from build123d import *

# Parameters (mm, degrees)
SKETCH_1_W             = 14
SKETCH_1_H             = 15
EXTRUDE_1_DEPTH        = 35
SKETCH_2_R             = 6
CUT_EXTRUDE_1_DEPTH    = 15
CUT_EXTRUDE_2_REACH    = 17
SKETCH_3_W             = 2
SKETCH_3_H             = 10
SKETCH_3_W_2           = 7
HOLE_WIZARD_M4_1_D     = 3.3
HOLE_WIZARD_M4_1_DEPTH = 5
SKETCH_4_R             = 4
CUT_EXTRUDE_3_DEPTH    = 1
FILLET_1_R             = 0.5


with BuildPart() as part:
    # 草图1 → 凸台-拉伸1 (new body)
    with BuildSketch(Plane.XY):
        with Locations((7, -7.5)):
            Rectangle(SKETCH_1_W, SKETCH_1_H)
    extrude(amount=EXTRUDE_1_DEPTH)

    # 草图2 → 切除-拉伸1 (cut)
    with BuildSketch(Plane.XY.offset(35)):
        with Locations((7, -7.5)):
            Circle(SKETCH_2_R)
    extrude(amount=-CUT_EXTRUDE_1_DEPTH, mode=Mode.SUBTRACT)

    # 草图3 → 切除-拉伸2 (cut, up to next)
    with BuildSketch(Plane.XZ.offset(15), mode=Mode.PRIVATE) as cut_extrude_2_sk1:
        with Locations((1, 5)):
            Rectangle(SKETCH_3_W, SKETCH_3_H)
    cut_extrude_2_tool1 = extrude(cut_extrude_2_sk1.sketch, amount=-CUT_EXTRUDE_2_REACH, mode=Mode.PRIVATE) & part.part
    add(cut_extrude_2_tool1.solids().sort_by_distance((1, -15, 5))[0], mode=Mode.SUBTRACT)
    # 草图3 → 切除-拉伸2 (cut, up to next)
    with BuildSketch(Plane.XZ.offset(15), mode=Mode.PRIVATE) as cut_extrude_2_sk2:
        with Locations((10.5, 5)):
            Rectangle(SKETCH_3_W_2, SKETCH_3_H)
    cut_extrude_2_tool2 = extrude(cut_extrude_2_sk2.sketch, amount=-CUT_EXTRUDE_2_REACH, mode=Mode.PRIVATE) & part.part
    add(cut_extrude_2_tool2.solids().sort_by_distance((10.5, -15, 5))[0], mode=Mode.SUBTRACT)

    # M4 螺纹孔1
    with Locations(Plane.ZY.offset(-2)):
        with Locations((5, -7.5)):
            Hole(HOLE_WIZARD_M4_1_D / 2, depth=HOLE_WIZARD_M4_1_DEPTH)

    # 草图4 → 切除-拉伸3 (cut)
    with BuildSketch(Plane.ZY.offset(-2)):
        with Locations((5, -7.5)):
            Circle(SKETCH_4_R)
    extrude(amount=-CUT_EXTRUDE_3_DEPTH, mode=Mode.SUBTRACT)

    # 圆角1
    fillet_1_edges = [part.edges().sort_by_distance(p)[0] for p in [
        (1, -7.5, 20),
        (1, -7.5, 35),
        (0, -7.5, 10),
        (14, -7.5, 10),
        (0, 0, 22.5),
        (14, 0, 22.5),
        (14, -15, 22.5),
        (0, -15, 22.5),
    ]]
    fillet(fillet_1_edges, radius=FILLET_1_R)


solid = part.part
Verification items for the finished model (mm, model axes). A direction names the side the tool comes from. Give positions to 0.01 mm unless a question says otherwise; leave off trailing zeros. Order: outer loops, then holes, each group sorted by start corner. A loop starts at its lowest first (then second) coordinate and runs counter-clockwise, first axis right, second up. Notation, with made-up numbers: (1.25, 70.25) -> (53.25, 70.25) arc R21 ccw to (53.25, 97.25) -> close; hole circle Ø10 at (64, 6.25). An arc over 180 degrees is marked (long way). Answer as CSV lines item,"result".
Q1. Sectioned sample at B-B on z = 24. Record the cut outline in (x, y), plus the area to 3 significant figures.
Solutions:
outline,"(0, -14.5) arc R0.5 ccw to (0.5, -15) -> (13.5, -15) arc R0.5 ccw to (14, -14.5) -> (14, -0.5) arc R0.5 ccw to (13.5, 0) -> (0.5, 0) arc R0.5 ccw to (0, -0.5) -> close; hole circle Ø12 at (7, -7.5)"
area,"96.7 mm²"
Q2. Release check for a two-part mould opening along Z. For faces 1 (the flat face through (3, -7, 7)), 2 (the flat face through (10, -8, 10)), 3 (the flat face through (7, 0, 21)) record: +Z half, -Z half, draft (parallel to the pull), parting line (faces both ways), or undercut.
Solutions:
face 1,"undercut"
face 2,"-Z half"
face 3,"draft"
Q3. Sectioned sample at A-A on y = -7.5. Record the cut outline in (x, z).
Solutions:
outline,"(0, 10.5) arc R0.5 ccw to (0.5, 10) -> (2, 10) -> (2, 9) -> (3, 9) -> (3, 6.65) -> (7, 6.65) -> (7, 10) -> (13.5, 10) arc R0.5 ccw to (14, 10.5) -> (14, 35) -> (13.5, 35) arc R0.5 ccw to (13, 34.5) -> (13, 20.5) arc R0.5 cw to (12.5, 20) -> (1.5, 20) arc R0.5 cw to (1, 20.5) -> (1, 34.5) arc R0.5 ccw to (0.5, 35) -> (0, 35) -> close; (2, 0) -> (7, 0) -> (7, 3.35) -> (3, 3.35) -> (3, 1) -> (2, 1) -> close"
Q4. Access from +Z, -Z, +X, -X, +Y, -Y to the whole of each face (thin tool, end or side, straight path). Record for faces 4 (the cylindrical face through (2.493, -6.299, 8.815)), 5 (the flat face through (7, -9.3, 4.9)), 6 (the flat face through (7, -7, 20)).
Solutions:
face 4,"-X"
face 5,"-Z, +X, +Y, -Y"
face 6,"+Z"
Q5. Depth check by flat-ended pin: pin 1 (4.5 mm diameter, centred on y = -7.5, z = 5, fed in from +X); pin 2 (1.7 mm diameter, centred on x = 1, y = -7, fed in from -Z); pin 3 (2.5 mm diameter, centred on y = -7, z = 6.5, fed in from -X). Enter the tip coordinate at first touch or a pass-through.
Solutions:
pin 1,"stops at x = 7"
pin 2,"stops at z = 10"
pin 3,"stops at x = 3"
Q6. Scan lines: probe 1 along Y at (x, z) = (3.75, 5); probe 2 along Y at (x, z) = (2.55, 5); probe 3 along Z at (x, y) = (12.25, -7.5). Record each from-to range of solid material in increasing order.
Solutions:
probe 1,"y = -15 to -9.15, -5.85 to 0"
probe 2,"y = -15 to -11.5, -3.5 to 0"
probe 3,"z = 10 to 20"
Q7. Sectioned sample at C-C on z = 5. Record the cut outline in (x, y).
Solutions:
outline,"(2, -15) -> (7, -15) -> (7, -9.15) -> (3, -9.15) -> (3, -11.5) -> (2, -11.5) -> close; (2, -3.5) -> (3, -3.5) -> (3, -5.85) -> (7, -5.85) -> (7, 0) -> (2, 0) -> close"
